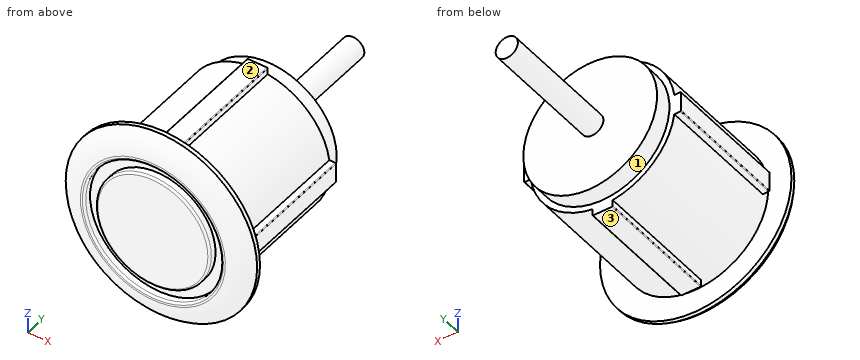
Autodesk Inventor part; units mm, degrees
ref_plane "YZ Plane" through (0, 0, 0) normal (1, 0, 0) x (0, 1, 0)
ref_plane "XZ Plane" through (0, 0, 0) normal (0, 1, 0) x (-1, 0, 0)
ref_plane "XY Plane" through (0, 0, 0) normal (0, 0, 1) x (1, 0, 0)
sketch "Skizze1" plane through (0, 0, 0) normal (0, 1, 0) x (-1, 0, 0)
  circle A0 centre (0, 0) radius 9
  dimension "d0" = 18
extrude "Extrusion1" add sketch "Skizze1" along normal blind 16.34
sketch "Skizze2" plane through (0, 16.34, 0) normal (0, 1, 0) x (1, 0, 0)
  circle A0 centre (0, 0) radius 8.3
  dimension "d3" = 16.6
extrude "Extrusion2" add sketch "Skizze2" along normal blind 2.16
sketch "Skizze3" plane through (0, 0, 0) normal (0, -1, 0) x (1, 0, 0)
  circle A0 centre (0, 0) radius 11.875
  dimension "d6" = 23.75
extrude "Extrusion3" add sketch "Skizze3" along normal blind 2
sketch "Skizze4" plane through (0, -2, 0) normal (0, -1, 0) x (1, 0, 0)
  circle A0 centre (0, 0) radius 7.075
  circle A1 centre (0, 0) radius 8.5
  dimension "d9" = 14.15
  dimension "d10" = 17
extrude "Extrusion4" cut sketch "Skizze4" against normal blind 1
fillet "Rundung1" radius 0.25 2 edges at (-7.075, -2, 0) (-8.5, -2, 0)
sketch "Skizze5" plane through (0, 0, 0) normal (1, 0, 0) x (0, 1, 0)
  line L0 (-2, 11.875) -> (-2, -11.875)
  line L1 (0, 11.875) -> (-2, 11.875)
  arc A0 (-0.5, 11.875) -> (-2, 8.9956) centre (1.5136, 8.9956) ccw
  line L2 (0, 0) -> (-4.6348, 0)
  dimension "d14" = 0.5
revolve "Umdrehung1" cut sketch "Skizze5" angle 360 about axis through (0, 0, 0) along (0, -1, 0)
sketch "Skizze6" plane through (0, 16.34, 0) normal (0, 1, 0) x (1, 0, 0)
  line L0 (-8.2456, -1.2678) -> (-9.7456, -1.2678)
  line L1 (-9.7456, -1.2678) -> (-9.7456, 1.2678)
  line L2 (-9.7456, 1.2678) -> (-8.2456, 1.2678)
  line L3 (-8.2456, 1.2678) -> (-8.2456, -1.2678)
  circle A0 centre (0, 0) radius 8.9956
  line L4 (-8.2456, -1.2678) -> (-9.7456, 1.2678) construction
  line L5 (-9.7456, -1.2678) -> (-8.2456, 1.2678) construction
  point P0 (-8.9956, 0)
  dimension "d16" = 0.75
extrude "Extrusion5" add sketch "Skizze6" against normal blind 15.5 contours L0 A0 L2 L3 | L0 L1 L2 A0 picked at (-8.4923, -0.1413)
fillet "Rundung2" radius 0.1 2 edges at (-9.7456, 8.59, -1.2678) (-9.7456, 8.59, 1.2678)
pattern_circular "Runde Anordnung1" count 4 over 360 about axis through (0, 0, 0) along (0, 1, 0) of "Extrusion5", "Rundung2"
sketch "Skizze7" plane through (0, 18.5, 0) normal (0, 1, 0) x (1, 0, 0)
  circle A0 centre (-0.2666, 0) radius 1.375
  point P0 (0, 0)
  dimension "d23" = 2.75
extrude "Extrusion6" add sketch "Skizze7" along normal blind 15
properties part number "JSN-SR04 US Sensor" material "ABS-Kunststoff"
Source: CAD feature listing. Evaluate the final solid. Frame: model axes, mm. Face numbers are marked on the shaded views. A direction names the side the tool comes from. Give positions to 0.01 mm unless a question says otherwise; leave off trailing zeros. Loops run counter-clockwise (first coordinate to the right, second up) from the corner with the lowest first, then second, coordinate; pieces in that order, holes last. Notation, with made-up numbers: (-4, 57) -> (38, 57) arc R6 ccw to (38, 68) -> close; hole circle Ø7 at (2.5, 55.25). An arc over 180 degrees is marked (long way). Use a Markdown table: item, result. Add a question column.
1) Section query D-D, the plane y = 23. Return the cut outline in (x, z) (3 decimals), then the cut area to 3 significant figures.
2) Section query B-B, the plane y = 8.5. Return the cut outline in (x, z).
3) First-contact query: pin 1 (2.5 mm diameter, centred on x = -0.5, y = 4.5, fed in from -Z); pin 2 (10 mm diameter, centred on x = 1.5, y = 8, fed in from +Z); pin 3 (8 mm diameter, centred on y = 14.5, z = 8.5, fed in from +X). Flat tips, straight axial feed; report the tip coordinate or a pass-through.
4) Reachability of the marked faces 1, 2 and 3 from +Z, -Z, +X, -X, +Y, -Y: full face, straight path, thin tool, end or side. Return the list, or none.
5) Line query: line 1 along Z through (x, y) = (0, -1.25) (3 decimals); line 2 along Y through (x, z) = (-0.75, -8.75); line 3 along Y through (x, z) = (3.75, -5). Output: solid intervals per line, ascending. Write a range as [from, to].
Numbers:
| question | item | result |
|---|---|---|
| 1 | outline | circle Ø2.75 at (-0.267, 0) |
| 1 | area | 5.94 mm2 |
| 2 | outline | (-9.75, -1.17) arc R0.1 ccw to (-9.65, -1.27) -> (-8.91, -1.27) arc R9 ccw to (-1.27, -8.91) -> (-1.27, -9.65) arc R0.1 ccw to (-1.17, -9.75) -> (1.17, -9.75) arc R0.1 ccw to (1.27, -9.65) -> (1.27, -8.91) arc R9 ccw to (8.91, -1.27) -> (9.65, -1.27) arc R0.1 ccw to (9.75, -1.17) -> (9.75, 1.17) arc R0.1 ccw to (9.65, 1.27) -> (8.91, 1.27) arc R9 ccw to (1.27, 8.91) -> (1.27, 9.65) arc R0.1 ccw to (1.17, 9.75) -> (-1.17, 9.75) arc R0.1 ccw to (-1.27, 9.65) -> (-1.27, 8.91) arc R9 ccw to (-8.91, 1.27) -> (-9.65, 1.27) arc R0.1 ccw to (-9.75, 1.17) -> close |
| 3 | pin 1 | stops at z = -9.75 |
| 3 | pin 2 | stops at z = 9.75 |
| 3 | pin 3 | stops at x = 7.79 |
| 4 | face 1 | +Y |
| 4 | face 2 | +Z, +X, -X, +Y |
| 4 | face 3 | -Z, +X, -X, +Y |
| 5 | line 1 | z = [-11.165, -8.5], [-7.075, 7.075], [8.5, 11.165] |
| 5 | line 2 | y = [-2, 16.34] |
| 5 | line 3 | y = [-2, 18.5] |
